Here's how the part is built. I have some questions about the finished solid (model axes, mm). Face numbers are marked on the shaded views. A direction names the side the tool comes from. Round coordinates to 2 decimals unless told otherwise and drop trailing zeros. Write each loop counter-clockwise with the first axis right and the second up, starting at its lowest first coordinate (ties: lowest second). Pieces come first, ordered by that corner, then holes. Notation, with made-up numbers: M -38,-9.75 L 5,-9.75 A18 cw 5,1.25 Z; hole C 20,40 d9. An arc over 180 degrees is marked long. Use a Markdown table: item, result. Add a question column.
```python
from build123d import *

# Parameters (mm, degrees)
ESQUISSE1_W             = 40
ESQUISSE1_H             = 62
BOSS_EXTRU_1_DEPTH      = 5
ESQUISSE2_W             = 20
ESQUISSE2_H             = 3.5
ENL_V_MAT_EXTRU_1_DEPTH = 6
ESQUISSE3_W             = 20
ESQUISSE3_H             = 3.5
ENL_V_MAT_EXTRU_2_DEPTH = 6
ESQUISSE8_W             = 3.1
ESQUISSE8_H             = 3
ESQUISSE8_H_2           = 5
ESQUISSE8_W_2           = 1.225
ENL_V_MAT_EXTRU_3_DEPTH = 6
ESQUISSE9_W             = 10
ESQUISSE9_H             = 65
BOSS_EXTRU_2_DEPTH      = 5
ESQUISSE10_R            = 1.05
ENL_V_MAT_EXTRU_4_DEPTH = 6


with BuildPart() as part:
    # Esquisse1 → Boss.-Extru.1 (new body)
    with BuildSketch(Plane.XY.offset(5)):
        Rectangle(ESQUISSE1_W, ESQUISSE1_H)
    extrude(amount=-BOSS_EXTRU_1_DEPTH)

    # Esquisse2 → Enlèv. mat.-Extru.1 (cut, through all)
    with BuildSketch(Plane(origin=(0, 0, 0), x_dir=(-1, 0, 0), z_dir=(0, 0, -1))):
        with Locations((0, 29.25)):
            Rectangle(ESQUISSE2_W, ESQUISSE2_H)
    extrude(amount=-ENL_V_MAT_EXTRU_1_DEPTH, mode=Mode.SUBTRACT)

    # Esquisse3 → Enlèv. mat.-Extru.2 (cut, through all)
    with BuildSketch(Plane(origin=(0, 0, 0), x_dir=(-1, 0, 0), z_dir=(0, 0, -1))):
        with Locations((0, -29.25)):
            Rectangle(ESQUISSE3_W, ESQUISSE3_H)
    extrude(amount=-ENL_V_MAT_EXTRU_2_DEPTH, mode=Mode.SUBTRACT)

    # Esquisse8 → Enlèv. mat.-Extru.3 (cut, through all)
    with BuildSketch(Plane.XY.offset(5)):
        with Locations((0, 21)):
            Rectangle(ESQUISSE8_W, ESQUISSE8_H)
        with Locations((0, 25)):
            Rectangle(ESQUISSE8_W, ESQUISSE8_H_2)
        with Locations((-2.1625, 21)):
            Rectangle(ESQUISSE8_W_2, ESQUISSE8_H)
        with Locations((2.1625, 21)):
            Rectangle(ESQUISSE8_W_2, ESQUISSE8_H)
        with Locations((0, 18)):
            Rectangle(ESQUISSE8_W, ESQUISSE8_H)
        with Locations((0, -18)):
            Rectangle(ESQUISSE8_W, ESQUISSE8_H)
        with Locations((-2.1625, -21)):
            Rectangle(ESQUISSE8_W_2, ESQUISSE8_H)
        with Locations((0, -21)):
            Rectangle(ESQUISSE8_W, ESQUISSE8_H)
        with Locations((2.1625, -21)):
            Rectangle(ESQUISSE8_W_2, ESQUISSE8_H)
        with Locations((0, -25)):
            Rectangle(ESQUISSE8_W, ESQUISSE8_H_2)
    extrude(amount=-ENL_V_MAT_EXTRU_3_DEPTH, mode=Mode.SUBTRACT)

    # Esquisse9 → Boss.-Extru.2 (add)
    with BuildSketch(Plane.XY.offset(5)):
        with Locations((-15, 0)):
            Rectangle(ESQUISSE9_W, ESQUISSE9_H)
        with Locations((15, 0)):
            Rectangle(ESQUISSE9_W, ESQUISSE9_H)
    extrude(amount=-BOSS_EXTRU_2_DEPTH)

    # Esquisse10 → Enlèv. mat.-Extru.4 (cut, through all)
    with BuildSketch(Plane(origin=(0, 0, 0), x_dir=(-1, 0, 0), z_dir=(0, 0, -1))):
        with Locations((-10.5, 10.5)):
            Circle(ESQUISSE10_R)
        with Locations((10.5, 10.5)):
            Circle(ESQUISSE10_R)
        with Locations((10.5, -2)):
            Circle(ESQUISSE10_R)
        with Locations((-10.5, -2)):
            Circle(ESQUISSE10_R)
    extrude(amount=-ENL_V_MAT_EXTRU_4_DEPTH, mode=Mode.SUBTRACT)


solid = part.part
```
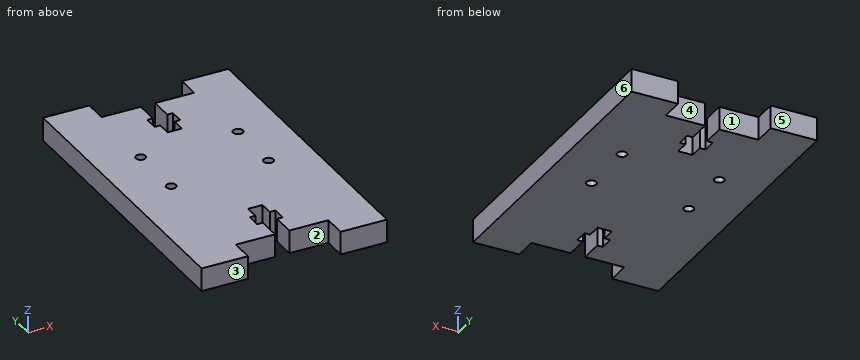
Item 1: I need wall thicknesses on probe 1 along Y at (x, z) = (-10.5, 1.45); probe 2 along Y at (x, z) = (2, 2.9); probe 3 along X at (y, z) = (21.5, 3) (3 decimals). Which ranges of each line are inside material? Lowest first, please. Write a range as from..to.
Item 2: On a 3-axis mill with a long thin cutter (end or side, diameter ignored), from which of +Z, -Z, +X, -X, +Y, -Y can I reach the whole of each face in a straight line? I mean the marked faces 1, 2 and 3. Say none if no direction works.
Item 3: If we mould it in two halves opening along X, with no side actions, what happens to the marked faces 4, 5 and 6? For each: +X half, -X half, draft (parallel to the pull), parting line (faces both ways), or undercut.
Item 4: For pin 1 Ø1.3 at (x, y) = (10.5, -2) entering from -Z; pin 2 Ø0.6 at (x, z) = (2, 3) entering from +Y, each with a flat end and sliding along its axis, tell me the tip position at first contact or that it passes through.
Item 5: Imagine slicing it at C-C on x = -3.5. List the corners of the cut face in (y, z) for me.
Item 6: Imagine slicing it at A-A on y = 10.5. List the corners of the cut face in (x, z) for me.
Item 7: Imagine slicing it at B-B on z = 2.9. Count the separate pieces of the cut face and the enclosed holes in it, plus the area to 3 significant figures.
The answers:
| question | item | result |
|---|---|---|
| 1 | probe 1 | -32.5..-3.05, -0.95..9.45, 11.55..32.5 |
| 1 | probe 2 | -27.5..-22.5, -19.5..19.5, 22.5..27.5 |
| 1 | probe 3 | -20..-2.775, 2.775..20 |
| 2 | face 1 | +Z, -Z, +Y |
| 2 | face 2 | +Z, -Z, -Y |
| 2 | face 3 | +Z, -Z, +X, -X, -Y |
| 3 | face 4 | undercut |
| 3 | face 5 | draft |
| 3 | face 6 | +X half |
| 4 | pin 1 | through |
| 4 | pin 2 | y = 27.5 |
| 5 | outline | M -27.5,0 L 27.5,0 L 27.5,5 L -27.5,5 Z |
| 6 | outline | M -20,0 L -11.55,0 L -11.55,5 L -20,5 Z; M -9.45,0 L 9.45,0 L 9.45,5 L -9.45,5 Z; M 11.55,0 L 20,0 L 20,5 L 11.55,5 Z |
| 7 | separate pieces | 1 |
| 7 | enclosed holes | 4 |
| 7 | area | 2,300 mm² |
